Source: CAD feature listing. Evaluate the final solid. Frame: model axes, mm. A direction names the side the tool comes from. Coordinates: 2 decimals unless noted, no trailing zeros. Loops run counter-clockwise (first coordinate to the right, second up) from the corner with the lowest first, then second, coordinate; pieces in that order, holes last. Notation, with made-up numbers: M -11.5,-4.75 L -7.5,-4.75 A10 ccw -7.5,14.25 Z; hole C 64.5,30 d4. An arc over 180 degrees is marked long. Write each question's results on one line, items separated by ' | '. Start each with the question number.
from build123d import *

# Parameters (mm, degrees)
F0_R     = 27.5
F1_DEPTH = 11
F2_R     = 23.5
F3_DEPTH = 8
F4_R     = 4
F4_R_2   = 3
F4_R_3   = 2.5
F5_DEPTH = 8


with BuildPart() as f1:
    # F0 (on Front) → F1 (new body)
    with BuildSketch(Plane.XZ):
        Circle(F0_R)
    extrude(amount=F1_DEPTH)

    # F2 (on face) → F3 (cut)
    with BuildSketch(Plane.XZ.offset(11)):
        Circle(F2_R)
    extrude(amount=-F3_DEPTH, mode=Mode.SUBTRACT)

    # F4 (on face) → F5 (join)
    with BuildSketch(Plane.XZ.offset(3)):
        with Locations((0, -10)):
            Circle(F4_R)
        with Locations((-17.5, 0)):
            Circle(F4_R_2)
        with Locations((17.5, 0)):
            Circle(F4_R_3)
    extrude(amount=F5_DEPTH)


solid = f1.part
Item 1: Cut plane C-C (z = -10). Output: boundary loops of the cut face in (x, y), then the cut area to 3 significant figures.
Item 2: Cut plane D-D (z = -1). Output: boundary loops of the cut face in (x, y), then the cut area to 3 significant figures.
Item 3: Mould query, pull axis X, two halves, no side actions, for faces 3 (the cylindrical face through (15, -7, 0)), 4 (the flat face through (17, -11, 0)), 5 (the cylindrical face through (-5.961, -5.423, -26.846)). Classes: +X half, -X half, draft (parallel to the pull), parting line (faces both ways), or undercut.
Item 4: Cut plane A-A (y = -4.5). Output: boundary loops of the cut face in (x, z), then the cut area to 3 significant figures.
Item 5: Access query for faces 1 (the flat face through (20.2, -11, 12.4)), 2 (the cylindrical face through (22.4, -7.1, 7.1)). Directions: +Z, -Z, +X, -X, +Y, -Y. A direction counts if a zero-diameter tool reaches every point of the face in a straight line with its end or side. Return the directions, or none.
Item 6: First-contact query: pin 1 Ø1 at (x, y) = (-16, -9) entering from -Z; pin 2 Ø1.5 at (x, y) = (-4, -4.5) entering from +Z; pin 3 Ø1.5 at (y, z) = (-1, 5) entering from +X. Flat tips, straight axial feed; report the tip coordinate or a pass-through.
Item 7: Cut plane B-B (x = 0). Output: boundary loops of the cut face in (y, z), then the cut area to 3 significant figures.
Item 8: Line query: probe 1 along Z at (x, y) = (0, -8); probe 2 along Z at (x, y) = (-1, -4.25); probe 3 along Y at (x, z) = (15, 8). Output: solid intervals per line, ascending.
Response values:
1) outline: M -25.62,-11 L -21.27,-11 L -21.27,-3 L -4,-3 L -4,-11 L 4,-11 L 4,-3 L 21.27,-3 L 21.27,-11 L 25.62,-11 L 25.62,0 L -25.62,0 Z | area: 287 mm2
2) outline: M -27.48,-11 L -23.48,-11 L -23.48,-3 L -20.33,-3 L -20.33,-11 L -14.67,-11 L -14.67,-3 L 15.21,-3 L 15.21,-11 L 19.79,-11 L 19.79,-3 L 23.48,-3 L 23.48,-11 L 27.48,-11 L 27.48,0 L -27.48,0 Z | area: 311 mm2
3) face 3: undercut | face 4: draft | face 5: parting line
4) outline: C 0,0 d55; C -17.5,0 d6; C 0,-10 d8; C 17.5,0 d5; hole C 0,0 d47 | area: 739 mm2
5) face 1: +Z, -Z, +X, -X, -Y | face 2: -Y
6) pin 1: stops at z = -22.72 | pin 2: stops at z = 27.31 | pin 3: stops at x = 27.17
7) outline: M -11,-27.5 L 0,-27.5 L 0,27.5 L -11,27.5 L -11,23.5 L -3,23.5 L -3,-6 L -11,-6 L -11,-14 L -3,-14 L -3,-23.5 L -11,-23.5 Z | area: 293 mm2
8) probe 1: z = -27.5 to -23.5, -14 to -6, 23.5 to 27.5 | probe 2: z = -27.48 to -23.48, -13.87 to -6.13, 23.48 to 27.48 | probe 3: y = -3 to 0
